Work out the finished part from the listing and answer in its coordinate system (mm). A direction names the side the tool comes from. Round coordinates to 2 decimals unless told otherwise and drop trailing zeros. Write each loop counter-clockwise with the first axis right and the second up, starting at its lowest first coordinate (ties: lowest second). Pieces come first, ordered by that corner, then holes.
1. Find section B-B (x = -71.5). Write down the section's boundary in (y, z).
2. Find section C-C (y = 0.85). Write down the section's boundary in (x, z).
3. Flat-ended cylindrical pins translate along their axes: pin 1 Ø1.5 at (y, z) = (1.5, -23) entering from -X; pin 2 Ø0.8 at (x, y) = (-121, -1) entering from -Z; pin 3 Ø0.8 at (x, z) = (-1, 1) entering from +Y. Find the tip coordinate at first contact, or state that the pin passes through.
4. Straight lines are drawn through the part: probe 1 along X at (y, z) = (-1.4, -13); probe 2 along Y at (x, z) = (-99.5, -23.5); probe 3 along X at (y, z) = (-1.15, -19). For each, find the intervals that lie inside material, in ascending order.
5. Determine the mould class of faces 4 (the face through (-114, 1.6, -16)), 5 (the face through (-61.347, 0.986, -29.733)), 6 (the face through (-121, -2, -15)) for opening direction Z: pulls with the +Z half, pulls with the -Z half, needs draft (parallel to the pull), parting line crosses it, or undercut.
6. Find section A-A (z = -24). Write down the section's boundary in (x, y).
7. A tool of negligible diameter and unlimited length cuts with its end or side. For faces 1 (the face through (-119, -1, -15)), 2 (the face through (-63, 2, -15)), 3 (the face through (-121, 1, -15)), from which of +Z, -Z, +X, -X, +Y, -Y can it reach the whole face along a straight path? Write none if from no direction.
```python
from build123d import *

# Parameters (mm, degrees)
SKETCH2_W           = 121
SKETCH2_H           = 29.819553929
BASE_EXTRUDE_DEPTH  = 2
DRAFT1_ANGLE        = 5
FILLET3_R           = 2.5
BOSS_EXTRUDE1_DEPTH = 1.5
BOSS_EXTRUDE2_DEPTH = 2
CUT_EXTRUDE3_DEPTH  = 0.4
CUT_EXTRUDE3_TAPER  = 3


with BuildPart() as part:
    # Sketch2 → Base-Extrude (new body)
    with BuildSketch(Plane(origin=(0, 0, 0), x_dir=(1, 0, 0), z_dir=(0, 1, 0))):
        with Locations((-60.5, 14.909776965)):
            Rectangle(SKETCH2_W, SKETCH2_H)
    extrude(amount=BASE_EXTRUDE_DEPTH)

    # Draft1
    draft1_faces = [part.faces().sort_by_distance(p)[0] for p in [
        (-60.5, 1, 0),
        (-60.5, 1, -29.819553929),
    ]]
    draft(draft1_faces, Plane.ZX, DRAFT1_ANGLE)

    # Fillet3
    # the kernel refuses this fillet: 2.5 mm, written as the material it takes off along each edge
    with BuildSketch(Plane(origin=(0, 2, 5.94874703), x_dir=(-1.5669991185737358e-12, -1.0, 0), z_dir=(0, 0, -1))) as fillet3_piece_1:
        with BuildLine():
            CenterArc((2.5, 2.449489743), FILLET3_R, 180, 78.463040967)
            Line((0, 2.449489743), (-0.05, 2.449489743))
            Line((-0.05, 2.449489743), (-0.05, 0))
            Line((-0.05, 0), (0, -0.05))
            ThreePointArc((0, -0.05), (1, -0.05), (1.99, -0.048989795))
            Line((1.99, -0.048989795), (2, 0))
        make_face()
    extrude(amount=41.717047988, mode=Mode.SUBTRACT)

    # Sketch3 → Boss-Extrude1 (add)
    with BuildSketch(Plane.XZ):
        with BuildLine():
            Line((0, 0.298935188), (0, -30.118489117))
            ThreePointArc((0, -30.118489117), (-0.408349934, -31.487795511), (-1.5, -32.409776964))
            Line((-1.5, -32.409776964), (-1.5, 2.590223036))
            ThreePointArc((-1.5, 2.590223036), (-0.408349934, 1.668241582), (0, 0.298935188))
        make_face()
    extrude(amount=BOSS_EXTRUDE1_DEPTH)

    # Sketch4 → Boss-Extrude2 (add)
    with BuildSketch(Plane.XZ):
        with BuildLine():
            Line((-120.25, -18.469776964), (-121.75, -18.469776964))
            ThreePointArc((-121.75, -18.469776964), (-122.633883476, -18.103660441), (-123, -17.219776964))
            Line((-123, -17.219776964), (-123, -12.599776964))
            ThreePointArc((-123, -12.599776964), (-122.633883476, -11.715893488), (-121.75, -11.349776964))
            Line((-121.75, -11.349776964), (-120.25, -11.349776964))
            ThreePointArc((-120.25, -11.349776964), (-119.366116524, -11.715893488), (-119, -12.599776964))
            Line((-119, -12.599776964), (-119, -17.219776964))
            ThreePointArc((-119, -17.219776964), (-119.366116524, -18.103660441), (-120.25, -18.469776964))
        make_face()
    extrude(amount=BOSS_EXTRUDE2_DEPTH)

    # Sketch5 → Cut-Extrude3 (cut)
    with BuildSketch(Plane(origin=(-217.927600689, 2, 0), x_dir=(1, 0, 0), z_dir=(0, -1, 0))):
        Polygon((105.927600689, -19.909776964), (111.427600689, -14.909776964), (105.927600689, -9.909776964), (98.427600689, -9.909776964), (98.427600689, -19.909776964), align=None)
    extrude(amount=CUT_EXTRUDE3_DEPTH, taper=CUT_EXTRUDE3_TAPER, mode=Mode.SUBTRACT)


solid = part.part
```
Worked answers:
1. outline: (0, -29.82) - (2, -29.64) - (2, -0.17) - (0, 0) - close
2. outline: (-121, -29.75) - (-0.35, -29.75) - (-0.35, -0.07) - (-121, -0.07) - close
3. pin 1: stops at x = -121
3. pin 2: stops at z = -18.47
3. pin 3: stops at y = 0
4. probe 1: x = -123 to -119, -1.5 to 0
4. probe 2: y = 0 to 2
4. probe 3: x = -1.5 to 0
5. face 4: undercut
5. face 5: pulls with the -Z half
5. face 6: needs draft
6. outline: (-121, 0) - (-1.5, 0) - (-1.5, -1.5) - (0, -1.5) - (0, 0) arc R2.5 ccw to (-2.45, 2) - (-121, 2) - close
7. face 1: +Z, -Z, -Y
7. face 2: +Z, -Z, +X, -X, +Y
7. face 3: +Z, -Z, -X, +Y
